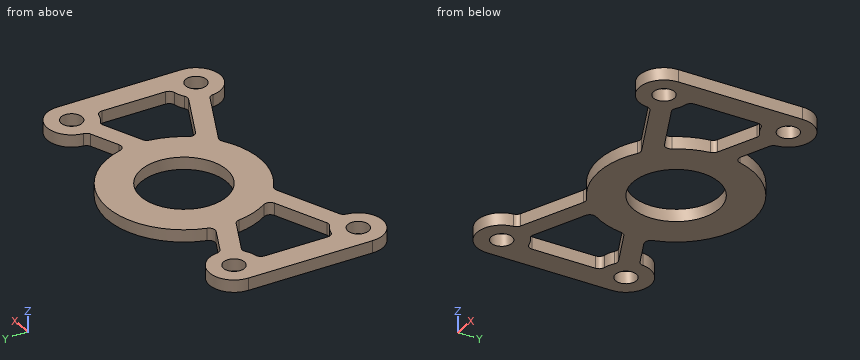
from build123d import *

# Parameters (mm, degrees)
SKETCH_1_R          = 12.5
EXTRUDE_1_DEPTH     = 2
SKETCH_1_R_2        = 4
EXTRUDE_1_2_DEPTH   = 2
EXTRUDE_1_3_DEPTH   = 2
EXTRUDE_1_4_DEPTH   = 2
EXTRUDE_1_5_DEPTH   = 2
EXTRUDE_2_DEPTH     = 2
EXTRUDE_3_DEPTH     = 2
FILLET_1_R          = 1
SKETCH_5_R          = 7
CUT_EXTRUDE_1_DEPTH = 33.668792448
HOLE_WIZARD_M3_1_D  = 3.4


with BuildPart() as part:
    # Sketch 1 → Extrude 1 (new body)
    with BuildSketch(Plane.XY):
        Circle(SKETCH_1_R)
    extrude(amount=EXTRUDE_1_DEPTH)



with BuildPart() as body_2:
    # Sketch 1 → Extrude 1 2 (new body)
    with BuildSketch(Plane.XY):
        with Locations((-22.5, 5)):
            Circle(SKETCH_1_R_2)
    extrude(amount=EXTRUDE_1_2_DEPTH)



with BuildPart() as body_3:
    # Sketch 1 → Extrude 1 3 (new body)
    with BuildSketch(Plane.XY):
        with Locations((-22.5, -15)):
            Circle(SKETCH_1_R_2)
    extrude(amount=EXTRUDE_1_3_DEPTH)


with BuildPart() as body_4:
    # Sketch 1 → Extrude 1 4 (new body)
    with BuildSketch(Plane.XY):
        with Locations((22.5, -15)):
            Circle(SKETCH_1_R_2)
    extrude(amount=EXTRUDE_1_4_DEPTH)


with BuildPart() as body_5:
    # Sketch 1 → Extrude 1 5 (new body)
    with BuildSketch(Plane.XY):
        with Locations((22.5, 5)):
            Circle(SKETCH_1_R_2)
    extrude(amount=EXTRUDE_1_5_DEPTH)


with BuildPart() as body_2_1:
    add(body_2.part)

    add(body_3.part)  # Extrude 2 merges body 3

    add(body_4.part)  # Extrude 2 merges body 4

    add(body_5.part)  # Extrude 2 merges body 5
    # Sketch 2 → Extrude 2 (add)
    with BuildSketch(Plane.XY.offset(2)):
        with BuildLine():
            Line((-26.5, 5), (-26.5, -15))
            ThreePointArc((-26.5, -15), (-25.328427125, -12.171572875), (-22.5, -11))
            Line((-22.5, -11), (-22.5, 1))
            ThreePointArc((-22.5, 1), (-25.328427125, 2.171572875), (-26.5, 5))
        make_face()
        with BuildLine():
            ThreePointArc((22.5, -11), (25.328427125, -12.171572875), (26.5, -15))
            Line((26.5, -15), (26.5, 5))
            ThreePointArc((26.5, 5), (25.328427125, 2.171572875), (22.5, 1))
            Line((22.5, 1), (22.5, -11))
        make_face()
    extrude(amount=-EXTRUDE_2_DEPTH)


with BuildPart() as part_1:
    add(part.part)

    add(body_2_1.part)  # Extrude 3 merges body 2
    # Sketch 3 → Extrude 3 (add, through all)
    with BuildSketch(Plane.XY.offset(2)):
        with BuildLine():
            ThreePointArc((-7.521060552, -9.984169879), (-8.74698669, -8.929738174), (-9.82653887, -7.725874309))
            Line((-9.82653887, -7.725874309), (-23.109207699, -13.629282677))
            ThreePointArc((-23.109207699, -13.629282677), (-23.870717323, -15.609207699), (-21.890792301, -16.370717323))
            Line((-21.890792301, -16.370717323), (-7.521060552, -9.984169879))
        make_face()
        with BuildLine():
            Line((23.109207699, -13.629282677), (9.82653887, -7.725874309))
            ThreePointArc((9.82653887, -7.725874309), (8.74698669, -8.929738174), (7.521060552, -9.984169879))
            Line((7.521060552, -9.984169879), (21.890792301, -16.370717323))
            ThreePointArc((21.890792301, -16.370717323), (23.870717323, -15.609207699), (23.109207699, -13.629282677))
        make_face()
        with BuildLine():
            Line((-12.319463678, 2.116793491), (-21.890792301, 6.370717323))
            ThreePointArc((-21.890792301, 6.370717323), (-23.870717323, 5.609207699), (-23.109207699, 3.629282677))
            Line((-23.109207699, 3.629282677), (-12.450816156, -1.107780231))
            ThreePointArc((-12.450816156, -1.107780231), (-12.489642096, 0.508763509), (-12.319463678, 2.116793491))
        make_face()
        with BuildLine():
            Line((21.890792301, 6.370717323), (12.319463678, 2.116793491))
            ThreePointArc((12.319463678, 2.116793491), (12.454784141, 1.06223915), (12.5, 0))
            ThreePointArc((12.5, 0), (12.487697986, -0.55443577), (12.450816156, -1.107780231))
            Line((12.450816156, -1.107780231), (23.109207699, 3.629282677))
            ThreePointArc((23.109207699, 3.629282677), (23.870717323, 5.609207699), (21.890792301, 6.370717323))
        make_face()
    extrude(amount=-EXTRUDE_3_DEPTH)

    # Fillet 1
    fillet_1_edges = [part_1.edges().sort_by_distance(p)[0] for p in [
        (12.319463678, 2.116793491, 1),
        (12.450816156, -1.107780231, 1),
        (-18.502288389, -14.864715584, 1),
        (-19.720703787, -12.123280938, 1),
        (-22.5, -11, 1),
        (-22.5, 1, 1),
        (7.521060552, -9.984169879, 1),
        (9.82653887, -7.725874309, 1),
        (19.720703787, -12.123280938, 1),
        (18.502288389, -14.864715584, 1),
        (22.5, -11, 1),
        (22.5, 1, 1),
        (-19.720703787, 2.123280938, 1),
        (-18.502288389, 4.864715584, 1),
        (-12.450816156, -1.107780231, 1),
        (-12.319463678, 2.116793491, 1),
        (-9.82653887, -7.725874309, 1),
        (-7.521060552, -9.984169879, 1),
        (18.502288389, 4.864715584, 1),
        (19.720703787, 2.123280938, 1),
    ]]
    fillet(fillet_1_edges, radius=FILLET_1_R)

    # Sketch 5 → Cut-Extrude 1 (cut, through all)
    with BuildSketch(Plane(origin=(0, 0, 0), x_dir=(-1, 0, 0), z_dir=(0, 0, -1))):
        Circle(SKETCH_5_R)
    extrude(amount=-CUT_EXTRUDE_1_DEPTH, mode=Mode.SUBTRACT)

    # Hole Wizard M3 _1 (through all)
    with Locations(Plane.XY.offset(2)):
        with Locations((-22.5, 5), (-22.5, -15), (22.5, -15), (22.5, 5)):
            Hole(HOLE_WIZARD_M3_1_D / 2)


solid = part_1.part
Verification items for the finished model (mm, model axes). Give positions to 0.01 mm unless a question says otherwise; leave off trailing zeros. Write each loop counter-clockwise with the first axis right and the second up, starting at its lowest first coordinate (ties: lowest second). Pieces come first, ordered by that corner, then holes.
(1) Gauge pin test, flat end, axial feed: pin 1 (12.5 mm diameter, centred on x = 0, y = 0, fed in from -Z). Record the tip position at first contact, or that the pin passes through.
(2) Cross-section at B-B (y = -7.5). Enter the section's corners in (x, z), plus the area to 3 significant figures.
(3) Cross-section at D-D (x = -9). Enter the section's corners in (y, z).
(4) Cross-section at C-C (z = 0.6). State how many separate pieces and enclosed holes the cut face has, plus the area to 3 significant figures.
(5) Cross-section at A-A (x = 0). Enter the section's corners in (y, z).
(6) Material ranges on line 1 (X direction, y = -3, z = 1.7); line 2 (Y direction, x = 19, z = 1.6); line 3 (Y direction, x = 16, z = 0.85), recorded low to high.
Worked out:
1. pin 1: passes through
2. outline: (-26.5, 0) - (-22.5, 0) - (-22.5, 2) - (-26.5, 2) - close; (-10.37, 0) - (10.37, 0) - (10.37, 2) - (-10.37, 2) - close; (22.5, 0) - (26.5, 0) - (26.5, 2) - (22.5, 2) - close
2. area: 57.5 mm2
3. outline: (-10.64, 0) - (8.67, 0) - (8.67, 2) - (-10.64, 2) - close
4. separate pieces: 1
4. enclosed holes: 7
4. area: 723 mm2
5. outline: (-12.5, 0) - (-7, 0) - (-7, 2) - (-12.5, 2) - close; (7, 0) - (12.5, 0) - (12.5, 2) - (7, 2) - close
6. line 1: x = -26.5 to -22.5, -12.13 to -6.32, 6.32 to 12.13, 22.5 to 26.5
6. line 2: y = -16.94 to -11.8, 1.8 to 6.94
6. line 3: y = -13.75 to -10.47, 0.47 to 3.75
